Could you check a few things on this model? Use its own coordinates, in mm. A direction names the side the tool comes from. Round coordinates to 2 decimals unless told otherwise and drop trailing zeros. Loops run counter-clockwise (first coordinate to the right, second up) from the corner with the lowest first, then second, coordinate; pieces in that order, holes last. Notation, with made-up numbers: (-28.5, 51.25) -> (3.5, 51.25) arc R25 ccw to (3.5, 87.25) -> close; hole circle Ø8 at (22, 47.25). An arc over 180 degrees is marked (long way). One line per item, written item: value.
Autodesk Inventor part; units mm, degrees
ref_plane "Work Plane1" through (-37.6, 24, -25.6) normal (0, 1, 0) x (1, 0, 0)
ref_plane "YZ Plane" through (0, 0, 0) normal (1, 0, 0) x (0, 1, 0)
ref_plane "XZ Plane" through (0, 0, 0) normal (0, 1, 0) x (-1, 0, 0)
sketch "Sketch1" plane through (0, 0, 0) normal (0, 1, 0) x (-1, 0, 0)
  circle A0 centre (0, 0) radius 10.3
  circle A1 centre (0, 0) radius 13.3
  dimension "d0" = 20.6
  dimension "d1" = 3
extrude "Extrusion1" add sketch "Sketch1" along normal blind 25
sketch "Sketch2" plane through (0, 0, 0) normal (0, 0, 1) x (1, 0, 0)
  circle A0 centre (0, 4) radius 16
  line L0 (13.3, 25) -> (-13.3, 25)
  line L1 (0, 25) -> (0, 20)
  point P0 (0, 0)
  dimension "d4" = 32
  dimension "d5" = 5
extrude "Extrusion2" cut sketch "Sketch2" against normal through all both and the other way through all
sketch "Sketch4" plane through (0, 0, 0) normal (1, 0, 0) x (0, 1, 0)
  line L0 (20, 13.3) -> (25, 13.3)
  line L1 (25, 13.3) -> (40, 25.6)
  line L2 (40, 25.6) -> (55, 25.6)
  line L3 (55, 25.6) -> (55, 22.6)
  line L4 (55, 22.6) -> (40, 22.6)
  line L5 (25, 10.3) -> (25, -10.3)
  line L6 (40, 22.6) -> (25, 10.3)
  line L7 (0, 0) -> (85.2959, 0)
  line L8 (25, 13.3) -> (25, 10.3)
  line L9 (25, -13.3) -> (25, 13.3)
  point P0 (25, 0)
  dimension "d8" = 22.6
  dimension "d9" = 3
  dimension "d11" = 15
  dimension "d12" = 30
revolve "Revolution1" add sketch "Sketch4" angle 360 about axis through (0, 0, 0) along (0, 1, 0)
chamfer "Chamfer1" distance 1 angle 45 5 edges at (0, 40, -25.6) (0, 55, -22.6) (10.3, 16.2438, -0.0012) (9.4045, 25, -9.4045) (-9.4045, 25, 9.4045)
sketch "Sketch5" plane through (0, 0, 0) normal (0, 1, 0) x (-1, 0, 0)
  circle A0 centre (0, 0) radius 13.9341
  circle A1 centre (0, 0) radius 35.7982
  point P0 (0, 0)
extrude "Extrusion3" cut sketch "Sketch5" along normal blind 24 contours A0 | A1
sketch "Sketch6" plane through (0, 24, 0) normal (0, -1, 0) x (1, 0, 0)
  circle A0 centre (0, 0) radius 10.3
  circle A1 centre (0, 0) radius 13.3
extrude "Extrusion4" add sketch "Sketch6" along normal blind 10
sketch "Sketch7" plane through (0, 14, 0) normal (0, -1, 0) x (1, 0, 0)
  circle A0 centre (0, 0) radius 6.75
  circle A1 centre (0, 0) radius 13.3
  circle A2 centre (0, 0) radius 10.3
  dimension "d21" = 13.5
extrude "Extrusion5" add sketch "Sketch7" against normal blind 11 contours A1 | A2
fillet "Fillet1" radius 2 1 edges at (-6.75, 14, 0)
sketch "Sketch8" plane through (0, 55, 0) normal (0, 1, 0) x (1, 0, 0)
  circle A0 centre (0, 0) radius 22.8
  dimension "d28" = 45.6
extrude "Extrusion6" cut sketch "Sketch8" against normal blind 15
sketch "Sketch10" plane through (0, 55, 0) normal (0, 1, 0) x (1, 0, 0)
  line L0 (-37.6, 25.6) -> (37.6, 25.6)
  line L1 (37.6, 25.6) -> (37.6, 0)
  line L2 (37.6, 0) -> (-37.6, 0)
  line L3 (-37.6, 0) -> (-37.6, 25.6)
  circle A0 centre (0, 0) radius 25.6
  circle A1 centre (0, 0) radius 25.6
  point P0 (-25.6, 0)
  point P1 (25.6, 0)
  point P2 (0, 25.6)
  point P3 (25.6, 0)
  dimension "d34" = 12
  dimension "d35" = 12
extrude "Extrusion8" add sketch "Sketch10" against normal blind 14 contours L0 A0 L2 L3 | L0 L1 L2 A0
sketch "Sketch11" plane through (-37.6, 55, -25.6) normal (0, 1, 0) x (1, 0, 0)
  line L0 (0, -25.6) -> (12, -25.6)
  line L1 (75.2, 0) -> (0, 0)
  line L2 (12, -25.6) -> (0, 0)
  line L3 (0, 0) -> (0, -25.6)
  arc A0 (12, -25.6) -> (63.2, -25.6) centre (37.6, -25.6) ccw
  line L4 (12, -25.6) -> (0, -25.6)
  arc A1 (63.2, -25.6) -> (37.6, 0) centre (37.6, -25.6) ccw
  line L5 (63.2, -25.6) -> (75.2, 0)
  line L6 (63.2, -25.6) -> (75.2, -25.6)
  line L7 (63.2, -25.6) -> (75.2, -25.6)
  line L8 (75.2, 0) -> (75.2, -25.6)
  line L9 (75.2, -25.6) -> (75.2, 0)
extrude "Extrusion9" [suppressed]
sketch "Sketch12" plane through (0, 0, 0) normal (0, 0, 1) x (1, 0, 0)
  circle A0 centre (-31.1, 48) radius 4.75
  circle A1 centre (31.1, 48) radius 4.75
  line L0 (-37.6, 55) -> (-37.6, 41)
  line L1 (37.6, 55) -> (37.6, 41)
  line L2 (37.6, 41) -> (25.6, 41)
  point P0 (0, 0)
  dimension "d40" = 9.5
  dimension "d41" = 6.5
  dimension "d42" = 6.5
  dimension "d43" = 7
extrude "Extrusion10" [suppressed]
sketch "Sketch13" plane through (0, 0, -21.6) normal (0, 0, 1) x (1, 0, 0)
  arc A0 (-35.725, 46.9175) -> (-35.725, 49.0825) centre (-31.1, 48) ccw
  circle A1 centre (-31.1, 48) radius 2.75
  arc A2 (35.725, 49.0825) -> (35.725, 46.9175) centre (31.1, 48) ccw
  circle A3 centre (31.1, 48) radius 2.75
  point P0 (0, 0)
  dimension "d46" = 5.5
extrude "Extrusion11" [suppressed]
sketch "Sketch17" plane through (0, 14, 0) normal (0, -1, 0) x (1, 0, 0)
  circle A0 centre (0, 0) radius 10.9341
  circle A1 centre (0, 0) radius 13.9341
  dimension "d53" = 3
extrude "Extrusion12" cut sketch "Sketch17" against normal through all contours A0
sketch "Sketch18" plane through (0, 14, 0) normal (0, -1, 0) x (1, 0, 0)
  circle A0 centre (0, 0) radius 20.3
  circle A1 centre (0, 0) radius 13.3
  dimension "d56" = 7
extrude "Extrusion13" add sketch "Sketch18" against normal blind 3
chamfer "Chamfer3" distance 7 angle 45 1 edges at (-13.3, 17, 0)
ref_plane "Work Plane1" through (-37.6, 24, -25.6) normal (0, 1, 0) x (1, 0, 0)
sketch "Sketch20" plane through (-37.6, 24, -25.6) normal (0, 1, 0) x (1, 0, 0)
  circle A0 centre (20.6, -25.6) radius 3
  line L0 (20.6, -29.0641) -> (17.6, -27.3321)
  line L1 (17.6, -27.3321) -> (17.6, -23.8679)
  line L2 (17.6, -23.8679) -> (20.6, -22.1359)
  line L3 (20.6, -22.1359) -> (23.6, -23.8679)
  line L4 (23.6, -23.8679) -> (23.6, -27.3321)
  line L5 (23.6, -27.3321) -> (20.6, -29.0641)
  point P0 (37.6, -25.6)
  dimension "d64" = 6
  dimension "d65" = 17
extrude "Extrusion14" cut sketch "Sketch20" against normal blind 7
sketch "Sketch21" plane through (0, 14, 0) normal (0, -1, 0) x (1, 0, 0)
  circle A0 centre (-17, 0) radius 1.75
  point P0 (0, 0)
  dimension "d68" = 3.5
  dimension "d69" = 17
extrude "Extrusion15" cut sketch "Sketch21" against normal blind 10
pattern_circular "Circular Pattern1" count 6 over 360 about axis through (0, 47.5, 0) along (0, 1, 0) of "Extrusion15", "Extrusion14"
sketch "Sketch23" plane through (-37.6, 55, -25.6) normal (0, 1, 0) x (1, 0, 0)
  line L0 (75.2, 0) -> (0, 0)
  arc A0 (12, -25.6) -> (63.2, -25.6) centre (37.6, -25.6) ccw
  circle A1 centre (37.6, -25.6) radius 23.6
  circle A2 centre (37.6, -25.6) radius 22.8
  line L1 (63.2, -25.6) -> (75.2, -25.6)
  line L2 (75.2, -25.6) -> (75.2, 0)
  line L3 (0, 0) -> (0, -25.6)
  line L4 (0, -25.6) -> (12, -25.6)
sketch "Sketch24" plane through (-37.6, 55, -25.6) normal (0, 1, 0) x (1, 0, 0)
  circle A0 centre (37.6, -25.6) radius 23.6
  circle A1 centre (37.6, -25.6) radius 23.6
  circle A2 centre (37.6, -25.6) radius 22.8
  circle A3 centre (37.6, -25.6) radius 22.8
extrude "Extrusion16" add sketch "Sketch24" against normal blind 2
sketch "Sketch25" plane through (-37.6, 55, -25.6) normal (0, 1, 0) x (1, 0, 0)
  circle A0 centre (37.6, -25.6) radius 22.8
  line L0 (75.2, 0) -> (0, 0)
  arc A1 (12, -25.6) -> (63.2, -25.6) centre (37.6, -25.6) ccw
  line L1 (63.2, -25.6) -> (75.2, -25.6)
  line L2 (75.2, -25.6) -> (75.2, 0)
  line L3 (0, 0) -> (0, -25.6)
  line L4 (0, -25.6) -> (12, -25.6)
extrude "Extrusion17" add sketch "Sketch25" along normal blind 3
sketch "Sketch26" plane through (-37.6, 58, -25.6) normal (0, 1, 0) x (1, 0, 0)
  line L0 (11.9256, -25.6) -> (63.2, -25.6)
  line L1 (63.2, -25.6) -> (63.2, 25)
  line L2 (63.2, 25) -> (11.9256, 25)
  line L3 (11.9256, 25) -> (11.9256, -25.6)
  line L4 (75.2, 0) -> (0, 0)
  circle A0 centre (17.9256, 15) radius 2.75
  circle A1 centre (57.2, 15) radius 2.75
  line L5 (37.6, 0) -> (75.2, 0)
  line L6 (63.2, 0) -> (11.9256, 0)
  line L7 (0, 0) -> (37.6, 0)
  point P0 (37.6, -25.6)
  point P1 (11.9256, 0)
  point P2 (63.2, 0)
  dimension "d79" = 25
  dimension "d80" = 5.5
  dimension "d81" = 6
  dimension "d82" = 6
  dimension "d91" = 15
extrude "Extrusion18" add sketch "Sketch26" against normal up to surface (17 mm away) contours L3 L2 L1 L4
sketch "Sketch27" plane through (-37.6, 58, -25.6) normal (0, 1, 0) x (1, 0, 0)
  line L0 (11.9256, 25) -> (11.9256, 0)
  line L1 (-19.2052, -40.8404) -> (11.9256, -40.8404)
  line L2 (11.9256, -40.8404) -> (11.9256, 11.2059)
  line L3 (11.9256, 11.2059) -> (-19.2052, 11.2059)
  line L4 (-19.2052, 11.2059) -> (-19.2052, -40.8404)
  line L5 (63.2, 0) -> (63.2, 25)
  line L6 (63.2, 17.9527) -> (82.2369, 17.9527)
  line L7 (82.2369, 17.9527) -> (82.2369, -35.178)
  line L8 (82.2369, -35.178) -> (63.2, -35.178)
  line L9 (63.2, -35.178) -> (63.2, 17.9527)
  point P0 (37.6, -25.6)
extrude "Extrusion19" cut sketch "Sketch27" against normal through all
sketch "Sketch28" plane through (-37.6, 58, -25.6) normal (0, 1, 0) x (1, 0, 0)
  line L0 (20.6756, 12.25) -> (15.1756, 12.25)
  line L1 (15.1756, 12.25) -> (15.1756, 17.75)
  line L2 (15.1756, 17.75) -> (20.6756, 17.75)
  line L3 (20.6756, 17.75) -> (20.6756, 12.25)
  circle A0 centre (17.9256, 15) radius 2.75
  line L4 (20.6756, 12.25) -> (15.1756, 17.75) construction
  line L5 (15.1756, 12.25) -> (20.6756, 17.75) construction
  line L6 (59.95, 12.25) -> (54.45, 12.25)
  line L7 (54.45, 12.25) -> (54.45, 17.75)
  line L8 (54.45, 17.75) -> (59.95, 17.75)
  line L9 (59.95, 17.75) -> (59.95, 12.25)
  circle A1 centre (57.2, 15) radius 2.75
  line L10 (59.95, 12.25) -> (54.45, 17.75) construction
  line L11 (54.45, 12.25) -> (59.95, 17.75) construction
  circle A2 centre (17.9256, 12.25) radius 2.75
  circle A3 centre (17.9256, 17.75) radius 2.75
  circle A4 centre (57.2, 12.25) radius 2.75
  circle A5 centre (57.2, 17.75) radius 2.75
  point P0 (37.6, -25.6)
  point P1 (20.6756, 12.25)
  point P2 (20.6756, 17.75)
  dimension "d87" = 5.5
  dimension "d88" = 5.5
extrude "Extrusion20" cut sketch "Sketch28" against normal through all
sketch "Sketch29" plane through (0, 14, 0) normal (0, -1, 0) x (1, 0, 0)
  circle A0 centre (0, 0) radius 35.383
extrude "Extrusion21" cut sketch "Sketch29" against normal blind 10
sketch "Sketch31" plane through (0, 0, 0) normal (1, 0, 0) x (0, 1, 0)
  line L0 (24, 13.3) -> (25.7733, 13.9341)
  line L1 (24, 13.3) -> (19.5254, 11.7)
  line L2 (10.3519, 0) -> (30.0392, 0)
  line L3 (24, -13.3) -> (24, 13.3)
  line L4 (24, 11.7) -> (19.5254, 9.7)
  line L5 (19.5254, 11.7) -> (19.5254, 9.7)
  line L6 (24, 11.7) -> (24, 13.3)
  point P0 (0, 0)
  dimension "d95" = 11.7
  dimension "d96" = 2
revolve "Revolution2" add sketch "Sketch31" angle 360 about axis through (0, 10.3519, 0) along (0, 1, 0)
sketch "Sketch32" plane through (0, 19.5254, 0) normal (0, -1, 0) x (1, 0, 0)
  circle A0 centre (0, 0) radius 9.7
  circle A1 centre (0, 0) radius 11.7
extrude "Extrusion22" add sketch "Sketch32" along normal blind 10
sketch "Sketch33" plane through (-37.6, 58, -25.6) normal (0, 1, 0) x (1, 0, 0)
  circle A0 centre (37.6, -25.6) radius 22.65
  circle A1 centre (37.6, -25.6) radius 22.8
  circle A2 centre (37.6, -25.6) radius 22.8
  dimension "d100" = 45.3
extrude "Extrusion23" add sketch "Sketch33" against normal blind 18
fillet "Fillet2" radius 5 2 edges at (25.6, 49.5, -50.6) (-25.6744, 49.5, -50.6)
fillet "Fillet3" radius 1 1 edges at (-11.7, 9.5254, 0)
sketch "Sketch34" plane through (-37.6, 58, -25.6) normal (0, 1, 0) x (1, 0, 0)
  line L0 (-0.5139, -99.2858) -> (75.7139, -99.2858)
  line L1 (75.7139, -99.2858) -> (75.7139, 48.0858)
  line L2 (75.7139, 48.0858) -> (-0.5139, 48.0858)
  line L3 (-0.5139, 48.0858) -> (-0.5139, -99.2858)
  line L4 (-0.5139, -99.2858) -> (75.7139, 48.0858) construction
  line L5 (75.7139, -99.2858) -> (-0.5139, 48.0858) construction
  point P0 (37.6, -25.6)
extrude "Extrusion24" cut sketch "Sketch34" against normal blind 2.5
properties part number "Chute"
(1) If we section it at B-B, the plane y = 31: Please give me the cut outline in (x, z).
Recorded:
outline: circle Ø36.44 at (0, 0); hole circle Ø30.44 at (0, 0)
(2) If we section it at D-D, the plane y = 18.5: Please give me the cut outline in (x, z).
Recorded:
outline: circle Ø23.4 at (0, 0); hole circle Ø19.4 at (0, 0)
(3) If we section it at C-C, the plane z = -27.5: Please give me the cut outline in (x, y), then the cut area to 3 significant figures.
Recorded:
outline: (-25.67, 41) -> (25.6, 41) -> (25.6, 55.5) -> (-25.67, 55.5) -> close
area: 743 mm²
(4) I'm going to push flat-ended pins straight in: pin 1 Ø12 at (x, z) = (-5.5, -6.5) entering from +Y; pin 2 Ø2 at (x, y) = (13.5, 37.5) entering from -Z; pin 3 Ø2 at (x, y) = (-13, 30.5) entering from -Z; pin 4 Ø10 at (x, z) = (2, -2.5) entering from -Y. Where does each tip first touch, or does it pass through?
Recorded:
pin 1: y = 30.14
pin 2: z = -20.48
pin 3: z = -13.68
pin 4: through
(5) For faces 1 (the face through (19.7, 48.4, -46.1)), 2 (the face through (-4.91, 47.86, 22.11)), 3 (the face through (8, 24, -8)), 4 (the face through (-2.54, 15.09, 11.42)), which set-ups out of +Z, -Z, +X, -X, +Y, -Y let a thin tool reach every point of the face, with its end or its side?
Recorded:
face 1: +Y, -Y
face 2: +Y
face 3: none
face 4: -Y
(6) Thinking about a two-plate mould opening in X: for faces 5 (the face through (0.563, 48.148, 25.594)), 6 (the face through (-10.348, 26.663, 5.382)), 7 (the face through (0, 48, -50.6)), which applies, released by +X, released by -X, zero draft, split by the parting line, or undercut?
Recorded:
face 5: split by the parting line
face 6: undercut
face 7: zero draft
(7) If I drill on L1, parallel to Z at x = 0, y = 48.25; L2, parallel to X at y = 47, z = -40.5; L3, parallel to Z at x = 0, y = 16, over which ranges is the centre line in solid material (lowest first)?
Recorded:
L1: -50.6 to -22.65, 22.65 to 25.6
L2: -25.67 to -22.42, -16.92 to 16.85, 22.35 to 25.6
L3: -11.7 to -9.7, 9.7 to 11.7
(8) If we section it at A-A, the plane y = 50: Please give me the cut outline in (x, z).
Recorded:
outline: (-25.67, -45.6) arc R5 ccw to (-20.67, -50.6) -> (20.6, -50.6) arc R5 ccw to (25.6, -45.6) -> (25.6, 0) arc R25.6 ccw to (-25.6, 0) -> (-25.67, 0) -> close; hole circle Ø45.3 at (0, 0); hole (-22.42, -43.35) arc R2.75 ccw to (-16.92, -43.35) -> (-16.92, -37.85) arc R2.75 ccw to (-22.42, -37.85) -> close; hole (16.85, -43.35) arc R2.75 ccw to (22.35, -43.35) -> (22.35, -37.85) arc R2.75 ccw to (16.85, -37.85) -> close
